Autodesk Inventor part; units mm, degrees
ref_plane "YZ Plane" through (0, 0, 0) normal (1, 0, 0) x (0, 1, 0)
ref_plane "XZ Plane" through (0, 0, 0) normal (0, 1, 0) x (-1, 0, 0)
ref_plane "XY Plane" through (0, 0, 0) normal (0, 0, 1) x (1, 0, 0)
sketch "Sketch2" plane through (0, 0, 0) normal (0, 0, 1) x (1, 0, 0)
  line L0 (0, 0) -> (180, 0)
  line L1 (180, 0) -> (180, 220)
  line L2 (180, 220) -> (0, 220)
  line L3 (0, 220) -> (0, 0)
  dimension "d4" = 220
  dimension "d5" = 180
extrude "Extrusion2" add sketch "Sketch2" along normal blind 320
sketch "Sketch3" plane through (0, 220, 0) normal (0, 1, 0) x (1, 0, 0)
  line L0 (0, 0) -> (180, 0)
  line L1 (180, 0) -> (180, -320)
  line L2 (0, 0) -> (180, 0)
  line L3 (180, 0) -> (180, -120)
  line L4 (180, -120) -> (0, -120)
  line L5 (0, -120) -> (0, 0)
  dimension "d8" = 120
extrude "Extrusion3" add sketch "Sketch3" along normal blind 200
sketch "Sketch4" plane through (0, 0, 0) normal (0, -1, 0) x (1, 0, 0)
  line L0 (0, 0) -> (180, 0)
  line L1 (180, 0) -> (180, 320)
  line L2 (0, 0) -> (180, 0)
  line L3 (180, 0) -> (180, 320)
  line L4 (180, 320) -> (0, 320)
  line L5 (0, 320) -> (0, 0)
extrude "Extrusion4" add sketch "Sketch4" along normal blind 20
sketch "Sketch5" plane through (0, -20, 0) normal (0, -1, 0) x (1, 0, 0)
  line L0 (180, 320) -> (0, 320)
  line L1 (180, 120) -> (180, 0)
  line L2 (0, 320) -> (180, 320)
  line L3 (180, 320) -> (180, 0)
  line L4 (180, 0) -> (0, 0)
  line L5 (0, 0) -> (0, 320)
extrude "Extrusion5" add sketch "Sketch5" along normal blind 40
sketch "Sketch6" plane through (180, 220, 120) normal (1, 0, 0) x (0, 0, -1)
  line L0 (0, 0) -> (-200, 0)
  line L1 (-200, 0) -> (0, 0)
  line L2 (120, 200) -> (0, 200)
  line L3 (0, 0) -> (0, 200)
  line L4 (0, 200) -> (120, 200)
  line L5 (120, 200) -> (120, -280)
  line L6 (120, 200) -> (120, -280)
  line L7 (120, -280) -> (-200, -280)
  line L8 (120, -280) -> (-200, -280)
  line L9 (-200, -280) -> (-200, 0)
  point P0 (120, -220)
extrude "Extrusion6" add sketch "Sketch6" along normal blind 72
sketch "Sketch7" plane through (0, -60, 0) normal (0, -1, 0) x (1, 0, 0)
  line L0 (0, 0) -> (252, 0)
  line L1 (0, 320) -> (252, 320)
  line L2 (252, 320) -> (252, 0)
  line L3 (252, 0) -> (0, 0)
  line L4 (0, 0) -> (0, 320)
extrude "Extrusion7" cut sketch "Sketch7" against normal blind 40
sketch "Sketch8" plane through (0, -20, 0) normal (0, -1, 0) x (1, 0, 0)
  line L0 (0, 120) -> (0, 320)
  line L1 (0, 0) -> (252, 0)
  line L2 (0, 320) -> (252, 320)
  line L3 (252, 320) -> (252, 0)
  line L4 (252, 0) -> (0, 0)
  line L5 (0, 0) -> (0, 320)
extrude "Extrusion8" cut sketch "Sketch8" against normal blind 20
properties part number "Fuel tank newest"
Geometry: final body of the model. Coordinates: model frame, mm. A direction names the side the tool comes from. Give positions to 0.01 mm unless a question says otherwise; leave off trailing zeros. Order: outer loops, then holes, each group sorted by start corner. A loop starts at its lowest first (then second) coordinate and runs counter-clockwise, first axis right, second up. Notation, with made-up numbers: (-21, -37.5) -> (24, -37.5) arc R22 cw to (24, -14.5) -> close; hole circle Ø4 at (65, 68). An arc over 180 degrees is marked (long way). Answer as a JSON object with one key per item and string values.
Q1. Section A-A (x = 162.5). Output: boundary loops of the cut face in (y, z), plus the area to 3 significant figures.
Entries:
{"outline": "(0, 0) -> (420, 0) -> (420, 120) -> (220, 120) -> (220, 320) -> (0, 320) -> close", "area": "94,400 mm^2"}
Q2. Section B-B (y = 292.5). Output: boundary loops of the cut face in (x, z).
Entries:
{"outline": "(0, 0) -> (252, 0) -> (252, 120) -> (0, 120) -> close"}
Q3. Material intervals for probe 1 along Z at (x, y) = (64, 346.5); probe 2 along Y at (x, z) = (231, 270.5), sorted ascending.
Entries:
{"probe 1": "z = 0 to 120", "probe 2": "y = 0 to 220"}
Q4. Access query for faces 4 (the flat face through (124, 319, 120)), 5 (the flat face through (124, 420, 59)). Directions: +Z, -Z, +X, -X, +Y, -Y. A direction counts if a zero-diameter tool reaches every point of the face in a straight line with its end or side. Return the directions, or none.
Entries:
{"face 4": "+Z, +X, -X, +Y", "face 5": "+Z, -Z, +X, -X, +Y"}
Q5. Section C-C (z = 138). Output: boundary loops of the cut face in (x, y).
Entries:
{"outline": "(0, 0) -> (252, 0) -> (252, 220) -> (0, 220) -> close"}
Q6. Draft query along Z for faces 1 (the flat face through (124, 213, 0)), 2 (the flat face through (0, 166, 122)), 3 (the flat face through (124, 108, 320)). Return one class per face: released by +Z, released by -Z, zero draft, split by the parting line, or undercut.
Entries:
{"face 1": "released by -Z", "face 2": "zero draft", "face 3": "released by +Z"}
